```python
from build123d import *

# Parameters (mm, degrees)
F1_DEPTH  = 30
F2_R      = 5.05
F3_DEPTH  = 28.001
F4_W      = 16
F4_H      = 20
F4_R      = 5.05
F5_DEPTH  = 4
F7_R      = 11.1
F8_DEPTH  = 11.001
F9_SIZE   = 5
F10_R     = 2
F11_R     = 2.5
F12_DEPTH = 24.6047988697


with BuildPart() as f1:
    # F0 (on Front) → F1 (new body)
    with BuildSketch(Plane.XZ):
        with BuildLine():
            Line((-16, 0), (0, 0))
            Line((0, 0), (0, 9))
            Line((0, 9), (15, 25.6591877224))
            ThreePointArc((15, 25.6591877224), (7.8215314679, 27.9326389309), (0.3556593903, 26.9529731799))
            Line((0.3556593903, 26.9529731799), (-16, 21))
            Line((-16, 21), (-16, 0))
        make_face()
    extrude(amount=F1_DEPTH)

    # F2 (on face) → F3 (cut, through all)
    with BuildSketch(Plane(origin=(0, 0, 0), x_dir=(1, 0, 0), z_dir=(0, 0, -1))):
        with Locations((-8.4, 15)):
            Circle(F2_R)
    extrude(amount=-F3_DEPTH, mode=Mode.SUBTRACT)

    # F4 (on face) → F5 (cut)
    with BuildSketch(Plane(origin=(0, 0, 0), x_dir=(1, 0, 0), z_dir=(0, 0, -1))):
        with Locations((-8, 15)):
            Rectangle(F4_W, F4_H)
        with Locations((-8.4, 15)):
            Circle(F4_R, mode=Mode.SUBTRACT)
    extrude(amount=-F5_DEPTH, mode=Mode.SUBTRACT)

    # F7 (on offset) → F8 (cut, through all)
    with BuildSketch(Plane(origin=(0, 0, 17), x_dir=(1, 0, 0), z_dir=(0, 0, -1))):
        with Locations((-8.4, 15)):
            Circle(F7_R)
    extrude(amount=-F8_DEPTH, mode=Mode.SUBTRACT)

    # F9
    f9_edges = [f1.edges().sort_by_distance(p)[0] for p in [
        (-16, -30, 10.5),
        (-16, 0, 10.5),
    ]]
    chamfer(f9_edges, length=F9_SIZE)

    # F10
    f10_edges = [f1.edges().sort_by_distance(p)[0] for p in [
        (15, -15, 25.659188),
    ]]
    fillet(f10_edges, radius=F10_R)

    # F11 (on face) → F12 (cut, through all)
    with BuildSketch(Plane(origin=(-4.4753485292, 0, 4.0296219153), x_dir=(0, 1, 0), z_dir=(0.7431448255, 0, -0.6691306064))):
        with Locations((-22, 21.6883034293)):
            Circle(F11_R)
        with Locations((-8, 21.6883034293)):
            Circle(F11_R)
    extrude(amount=-F12_DEPTH, mode=Mode.SUBTRACT)


solid = f1.part
```
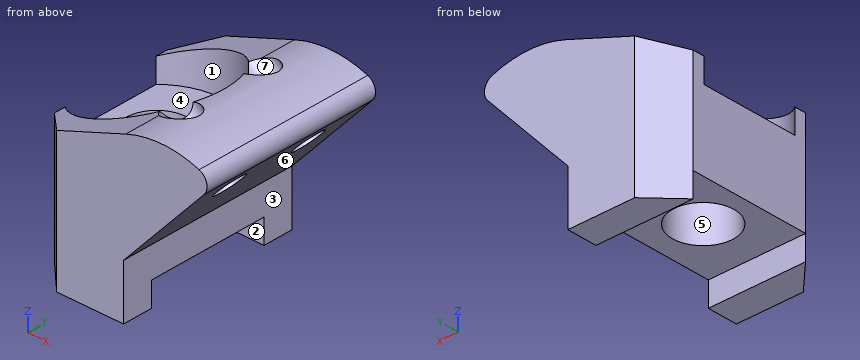
Model file for the job. Use its own axes, mm. Face numbers are marked on the shaded views. A direction names the side the tool comes from. Coordinates: 2 decimals unless noted, no trailing zeros. Loops run counter-clockwise (first coordinate to the right, second up) from the corner with the lowest first, then second, coordinate; pieces in that order, holes last. Notation, with made-up numbers: (57, 58.5) -> (116, 58.5) arc R24 ccw to (116, 90.5) -> close; hole circle Ø11 at (74.5, 85.25). An arc over 180 degrees is marked (long way). Answer as a JSON object with one key per item and string values.
Q1. Cut at A-A (y = -15). List the corners of the cut face in (x, z), and give its area (3 significant figures).
Report:
{"outline": "(-16, 4) -> (-13.45, 4) -> (-13.45, 17) -> (-16, 17) -> close; (-3.35, 4) -> (0, 4) -> (0, 9) -> (13.21, 23.67) arc R2 ccw to (12.43, 26.88) arc R17.36 ccw to (2.7, 27.62) -> (2.7, 17) -> (-3.35, 17) -> close", "area": "198 mm2"}
Q2. Probe probe 1 along Y at (x, z) = (-8.4, 11.25); probe 2 along X at (y, z) = (-15, 8); probe 3 along Z at (x, y) = (-6.5, -23.5). List the from-to ranges inside material, lowest first.
Report:
{"probe 1": "y = -30 to -20.05, -9.95 to 0", "probe 2": "x = -16 to -13.45, -3.35 to 0", "probe 3": "z = 4 to 17"}
Q3. Cut at D-D (y = -27). List the corners of the cut face in (x, z), and give its area (3 significant figures).
Report:
{"outline": "(-14, 0) -> (0, 0) -> (0, 9) -> (13.21, 23.67) arc R2 ccw to (12.43, 26.88) arc R17.36 ccw to (0.36, 26.95) -> (-14, 21.73) -> close", "area": "489 mm2"}
Q4. Pull direction Z, two halves, no side cores. Call the marked faces 4, 5, 6 and 7: released by +Z, released by -Z, zero draft, split by the parting line, or undercut.
Report:
{"face 4": "released by +Z", "face 5": "zero draft", "face 6": "released by -Z", "face 7": "undercut"}
Q5. 3-axis set-ups, long thin cutter, end or side, ignore diameter. For the marked faces 1, 2 and 3: which of +Z, -Z, +X, -X, +Y, -Y reach the whole face in a straight line?
Report:
{"face 1": "+Z", "face 2": "-Z, +X, -X", "face 3": "-Z, +X, +Y, -Y"}
Q6. Cut at B-B (z = 5.75). List the corners of the cut face in (x, y).
Report:
{"outline": "(-16, -25) -> (-11, -30) -> (0, -30) -> (0, 0) -> (-11, 0) -> (-16, -5) -> close; hole circle Ø10.1 at (-8.4, -15)"}
Q7. Flat gauge pins, fed straight in: P1, Ø4, axis at x = -7, z = 25, coming from the +Y side; P2, Ø10, axis at y = -12.5, z = 3, coming from the +X side; P3, Ø2, axis at y = -23, z = 13, coming from the +X side; P4, Ø2, axis at x = -10.5, y = -5.5, coming from the +Z side. Where does each tip first touch, or does it go through?
Report:
{"P1": "stops at y = 0", "P2": "stops at x = 0", "P3": "stops at x = 4.5", "P4": "stops at z = 17"}
Q8. Cut at C-C (x = -8.4). List the corners of the cut face in (y, z).
Report:
{"outline": "(-30, 0) -> (-25, 0) -> (-25, 4) -> (-20.05, 4) -> (-20.05, 17) -> (-26.1, 17) -> (-26.1, 23.77) -> (-30, 23.77) -> close; (-9.95, 4) -> (-5, 4) -> (-5, 0) -> (0, 0) -> (0, 23.77) -> (-3.9, 23.77) -> (-3.9, 17) -> (-9.95, 17) -> close"}
